Autodesk Inventor part; units mm, degrees
ref_plane "YZ Plane" through (0, 0, 0) normal (1, 0, 0) x (0, 1, 0)
ref_plane "XZ Plane" through (0, 0, 0) normal (0, 1, 0) x (-1, 0, 0)
ref_plane "XY Plane" through (0, 0, 0) normal (0, 0, 1) x (1, 0, 0)
sketch "スケッチ1" plane through (0, 0, 0) normal (0, 0, 1) x (1, 0, 0)
  line L0 (0, 0) -> (0, 40)
  line L1 (0, 40) -> (0, 190)
  line L2 (0, 40) -> (-45, 40)
  line L3 (0, 0) -> (-40, 0)
  spline S0 degree 2 poles (-40, 0) (-61.343, 41.3687) (0, 190) knots 0 0 0 1 1 1
  point P0 (0, 100)
  dimension "d0" = 40
  dimension "d1" = 150
  dimension "d2" = 45
  dimension "d3" = 40
  dimension "d14" = 100
revolve "回転1" add sketch "スケッチ1" angle 360 about axis through (0, 40, 0) along (0, 1, 0)
sketch "スケッチ4" plane through (0, 0, 0) normal (0, -1, 0) x (1, 0, 0)
  circle A0 centre (0, 0) radius 40
  line L0 (-30, -26.4575) -> (-30, 26.4575)
  circle A1 centre (0, 0) radius 50.9747
  line L1 (-30, -41.2119) -> (-30, 41.2119)
  point P0 (-30, 0)
  point P1 (-40, 0)
  dimension "d15" = 30
extrude "押し出し3" cut sketch "スケッチ4" against normal blind 400 contours L0 A0 | A0 L1 A1 picked at (-33.2623, -1.3742) picked at (-32.3949, 34.1789)
sketch "スケッチ5" plane through (-30, 0, -26.4575) normal (-1, 0, 0) x (0, 0, 1)
  line L0 (52.915, 0) -> (0, 0)
  point P0 (26.4575, 0)
  point P1 (26.4575, 0)
  point P2 (16.4575, 100)
  point P3 (16.4575, 130)
  point P4 (36.4575, 100)
  point P5 (36.4575, 130)
  dimension "d20" = 30
hole "穴1" at (-30, 100, -10) at (-30, 130, -10) at (-30, 130, 10) at (-30, 100, 10) direction (1, 0, 0) diameter 2.6 depth 40
sketch "スケッチ6" plane through (0, 0, 0) normal (0, -1, 0) x (1, 0, 0)
  circle A0 centre (-125, 0) radius 125
  point P0 (0, 0)
  dimension "d28" = 250
  dimension "d29" = 125
extrude "押し出し4" cut sketch "スケッチ6" against normal blind 400
sketch "スケッチ7" plane through (0, 0, 0) normal (0, -1, 0) x (1, 0, 0)
  circle A0 centre (0, 0) radius 32.5
  dimension "d32" = 65
extrude "押し出し5" cut sketch "スケッチ7" against normal blind 70
fillet "フィレット2" radius 7 1 edges at (32.5, 70, 0)
properties part number "newleg" material "ゴム、黒"
Design review of the part built by this model. Coordinates are the model's own, in mm. A direction names the side the tool comes from. Round coordinates to 2 decimals unless told otherwise and drop trailing zeros. Answer as CSV lines item,"result". Start each with the question number.
1) Wall thickness on line 1 along Z through (x, y) = (2.5, 100); line 2 along Z through (x, y) = (5.25, 130); line 3 along Y through (x, z) = (2, 10): over which ranges is each line inside the solid? List them lowest first. Write a range as [from, to].
2) For pin 1 Ø1.3 at (y, z) = (130, 10.5) entering from -X; pin 2 Ø2 at (y, z) = (130, -9.5) entering from -X; pin 3 Ø1 at (y, z) = (77.5, -34.5) entering from +X, all flat-tipped, find the tip position at first contact; note any pin that passes through.
3) Tool access review of faces 1 (the face through (11, 70, 0)), 2 (the face through (32.4, 0, -5.7)), 3 (the face through (32.49, 31.06, -0.77)): name each direction out of +Z, -Z, +X, -X, +Y, -Y from which nothing blocks a thin tool from reaching the whole face with its end or side.
Resolved:
1,line 1,"[-32.45, -11.3], [-8.7, 8.7], [11.3, 32.45]"
1,line 2,"[-22.31, -11.3], [-8.7, 8.7], [11.3, 22.31]"
1,line 3,"[70, 98.7], [101.3, 128.7], [131.3, 164.56]"
2,pin 1,"x = 10"
2,pin 2,"x = -0.33"
2,pin 3,"x = 18.25"
3,face 1,"-X, -Y"
3,face 2,"+Z, -Z, +X, -X, -Y"
3,face 3,"-Y"
